The listing builds one solid part. Answer for the finished solid, in the listing's coordinates (mm). Face numbers are marked on the shaded views. A direction names the side the tool comes from. Round coordinates to 2 decimals unless told otherwise and drop trailing zeros. Order: outer loops, then holes, each group sorted by start corner. A loop starts at its lowest first (then second) coordinate and runs counter-clockwise, first axis right, second up. Notation, with made-up numbers: (80, 0.5) -> (120, 0.5) arc R20 ccw to (120, 35.5) -> close; hole circle Ø3 at (30.25, 45). An arc over 180 degrees is marked (long way). Answer in a Markdown table with one row per item. Add a question column.
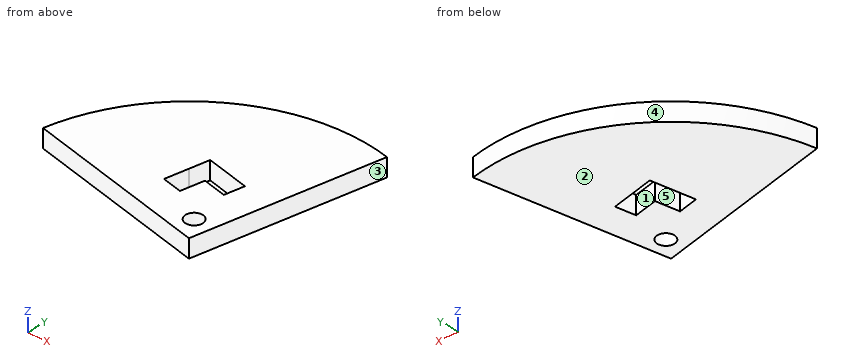
```python
from build123d import *

# Parameters (mm, degrees)
BOSS_EXTRUDE2_DEPTH = 3.81
SKETCH3_R           = 1.778
CUT_EXTRUDE1_DEPTH  = 83.609172725
CUT_EXTRUDE2_DEPTH  = 83.609172725


with BuildPart() as part:
    # Sketch2 → Boss-Extrude2 (new body)
    with BuildSketch(Plane.XY):
        with BuildLine():
            Line((-11.22087151, 59.495333804), (-19.039557078, 22.20621802))
            Line((-19.039557078, 22.20621802), (-56.328672862, 30.024903588))
            ThreePointArc((-56.328672862, 30.024903588), (-39.878298128, 54.102250241), (-11.22087151, 59.495333804))
        make_face()
    extrude(amount=BOSS_EXTRUDE2_DEPTH)

    # Sketch3 → Cut-Extrude1 (cut, through all)
    with BuildSketch(Plane.XY.offset(3.81)):
        with Locations((-21.986600099, 26.716998155)):
            Circle(SKETCH3_R)
    extrude(amount=-CUT_EXTRUDE1_DEPTH, mode=Mode.SUBTRACT)

    # Sketch4 → Cut-Extrude2 (cut, through all)
    with BuildSketch(Plane(origin=(0, 0, 0), x_dir=(-1, 0, 0), z_dir=(0, 0, -1))):
        Polygon((31.084073207, 40.641701891), (22.213000878, 38.781638338), (23.046994005, 34.804132654), (31.918066334, 36.664196207), align=None)
        Polygon((32.908433172, 31.940908208), (31.918066334, 36.664196207), (27.854066334, 35.812067175), (28.844433172, 31.088779176), align=None)
    extrude(amount=-CUT_EXTRUDE2_DEPTH, mode=Mode.SUBTRACT)


solid = part.part
```
1. The part is cut by section D-D (x = -48). Give the vertices of the cut face in (y, z), then the cut area to 3 significant figures.
2. The mould has two halves that part along Y. Classify the marked faces 3, 4 and 5: released by +Y, released by -Y, zero draft, split by the parting line, or undercut.
3. Straight lines are drawn through the part: line 1 along X through (y, z) = (37, 0.85); line 2 along X through (y, z) = (32, 1.5); line 3 along Y through (x, z) = (-29.5, 2.05). For each, find the intervals that lie inside material, in ascending order.
4. The part is cut by section B-B (y = 26). Give the vertices of the cut face in (x, z).
5. The part is cut by section C-C (x = -30.5). Give the vertices of the cut face in (y, z).
6. The part is cut by section A-A (z = 2.75). Give the vertices of the cut face in (x, y), then the cut area to 3 significant figures.
7. For the marked faces 1 and 2, determine the directions among +Z, -Z, +X, -X, +Y, -Y from which every point of the face is accessible in a straight line to the end or side of a thin tool.
8. Each of these flat-tipped pins is pushed along its axis until it touches: pin 1 (1 mm diameter, centred on x = -17.5, z = 2.5, fed in from +Y); pin 2 (2 mm diameter, centred on y = 53, z = 0.5, fed in from +X). Where does it stop, or does it pass through?
Report:
| question | item | result |
|---|---|---|
| 1 | outline | (28.28, 0) -> (46.96, 0) -> (46.96, 3.81) -> (28.28, 3.81) -> close |
| 1 | area | 71.2 mm^2 |
| 2 | face 3 | released by -Y |
| 2 | face 4 | released by +Y |
| 2 | face 5 | undercut |
| 3 | line 1 | x = -54.15 to -31.85, -22.59 to -15.94 |
| 3 | line 2 | x = -55.86 to -32.9, -28.65 to -16.99 |
| 3 | line 3 | y = 24.4 to 31.23, 40.31 to 58.84 |
| 4 | outline | (-37.13, 0) -> (-23.61, 0) -> (-23.61, 3.81) -> (-37.13, 3.81) -> close; (-20.36, 0) -> (-18.24, 0) -> (-18.24, 3.81) -> (-20.36, 3.81) -> close |
| 5 | outline | (24.61, 0) -> (31.44, 0) -> (31.44, 3.81) -> (24.61, 3.81) -> close; (40.52, 0) -> (58.54, 0) -> (58.54, 3.81) -> (40.52, 3.81) -> close |
| 6 | outline | (-56.33, 30.02) -> (-19.04, 22.21) -> (-11.22, 59.5) arc R38.1 ccw to start; hole (-32.91, 31.94) -> (-28.84, 31.09) -> (-27.85, 35.81) -> (-23.05, 34.8) -> (-22.21, 38.78) -> (-31.08, 40.64) -> close; hole circle Ø3.56 at (-21.99, 26.72) |
| 6 | area | 1,070 mm^2 |
| 7 | face 1 | +Z, -Z |
| 7 | face 2 | -Z, +X, -X, +Y, -Y |
| 8 | pin 1 | stops at y = 60.29 |
| 8 | pin 2 | stops at x = -12.37 |
